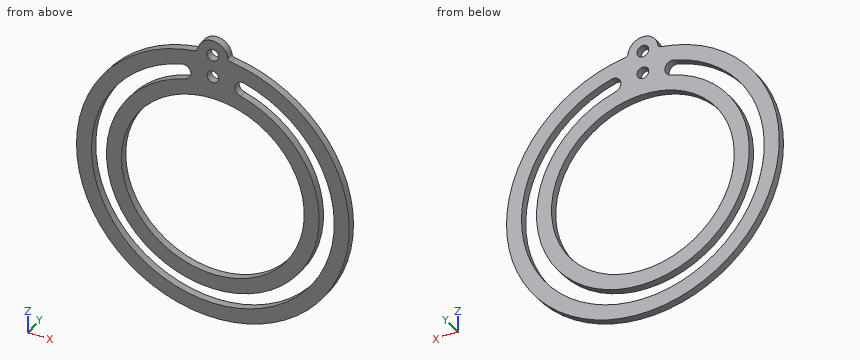
Autodesk Inventor part; units mm, degrees
ref_plane "YZ Plane" through (0, 0, 0) normal (1, 0, 0) x (0, 1, 0)
ref_plane "XZ Plane" through (0, 0, 0) normal (0, 1, 0) x (-1, 0, 0)
ref_plane "XY Plane" through (0, 0, 0) normal (0, 0, 1) x (1, 0, 0)
sketch "Sketch1" plane through (0, 0, 0) normal (0, 1, 0) x (-1, 0, 0)
  arc A0 (-9.3914, 47.3099) -> (9.3914, 47.3099) centre (0, 0) ccw
  arc A1 (-11.6619, 43.5227) -> (11.6619, 43.5227) centre (0, 0) ccw
  arc A2 (-13.3054, 49.6564) -> (13.3054, 49.6564) centre (0, 0) ccw
  circle A3 centre (0, 0) radius 38.708
  circle A4 centre (12.4836, 46.5895) radius 3.175
  circle A5 centre (-12.4836, 46.5895) radius 3.175
  line L0 (0, 0) -> (12.4836, 46.5895)
  line L1 (0, 0) -> (-12.4836, 46.5895)
  line L2 (0, 0) -> (0, 57.758)
  arc A6 (6.2927, 58.6092) -> (-6.2927, 58.6092) centre (0, 57.758) ccw
  arc A7 (6.2927, 58.6092) -> (7.6555, 57.2484) centre (7.8659, 58.8219) ccw
  arc A8 (-7.6555, 57.2484) -> (-6.2927, 58.6092) centre (-7.8659, 58.8219) ccw
  arc A9 (-7.6555, 57.2484) -> (7.6555, 57.2484) centre (0, 0) ccw
  point P0 (0, 48.233)
  point P1 (11.6619, 43.5227)
  point P2 (-11.6619, 43.5227)
  dimension "d0" = 96.4661
  dimension "d1" = 3.175
  dimension "d2" = 3.175
  dimension "d3" = 6.35
  dimension "d5" = 6.35
  dimension "d6" = 6.35
  dimension "d9" = 15
  dimension "d10" = 15
  dimension "d11" = 12.7
  dimension "d12" = 3.175
  dimension "d13" = 3.175
  dimension "d14" = 6.35
  dimension "d15" = 57.758
  dimension "d16" = 9.525
extrude "Extrusion1" add sketch "Sketch1" along normal blind 3.175 contours L1 A3 L0 A1 | A7 A9 A8 A6
hole "Hole1" at (0, 0, 48.233) at (0, 0, 57.758) direction (0, 1, 0) diameter 4.9784 end through all
equation "\"d0\" = ringDiam"
equation "\"d9\" = stageAngle"
equation "\"d10\" = stageAngle"
equation "\"d11\" = thickness"
equation "\"height\" = 203.2"
equation "\"thickness\" = 12.7"
equation "\"shaftDiam\" = 6.35"
equation "\"shaftSpace\" = 1.5875"
equation "\"stageSpace\" = 2.54"
equation "\"stageAngle\" = 15deg"
equation "\"bearingDiam\" = 9.5504"
equation "\"FlangeDiam\" = 12.7"
equation "\"FlangeDepth\" = 1.5875"
equation "\"smallFilet\" = 0.39687"
equation "\"ringDiam\" = 96.46608"
equation "\"stockHeight\" = 50.8"
equation "\"stockWidth\" = 76.2"
equation "\"stockRad\" = 9.525"
equation "\"stockGuage\" = 3.175"
equation "\"groundActu\" = 304.8"
equation "\"baseWidth\" = 1066.8"
equation "\"baseDepth\" = 254"
equation "\"capThickness\" = 3.175"
equation "\"sup1Len\" = 660.4"
equation "\"sup1Ang\" = 22.619865deg"
equation "\"sup2Len\" = 2079.37366"
equation "\"sup2Ang\" = 8.959949deg"
equation "\"supVertLen\" = 955.13561"
equation "\"supSideLen\" = 1531.12879"
equation "\"supSideAng\" = 19.376933deg"
properties part number "lock ring 2" material "Aluminum 6061"
Geometry: final body of the model. Coordinates: model frame, mm. Round coordinates to 2 decimals unless told otherwise and drop trailing zeros. Write each loop counter-clockwise with the first axis right and the second up, starting at its lowest first coordinate (ties: lowest second). Pieces come first, ordered by that corner, then holes.
Item 1: Pin query (flat end, axial travel): P1, Ø2, axis at x = -23, z = -28, coming from the +Y side; P2, Ø1.5, axis at x = 39, y = 1, coming from the +Z side. Return the tip coordinate at first contact, or that it passes through.
Item 2: Section query C-C (x = -15). Return loops of the section in (y, z) (3 decimals), plus the area to 3 significant figures.
Item 3: Section query B-B (x = 0). Return loops of the section in (y, z) (3 decimals), plus the area to 3 significant figures.
Item 4: Section query A-A (z = 0). Return loops of the section in (x, y) (3 decimals), plus the area to 3 significant figures.
Item 5: Section query D-D (y = 2.3). Give the number of separate pieces and of enclosed holes in the cut face, plus the area to 3 significant figures.
Item 6: Material intervals for L1, parallel to X at y = 1.55, z = 0; L2, parallel to Z at x = 1.5, y = 0.5; L3, parallel to X at y = 2.9, z = -21.5, sorted ascending.
Completed:
1. P1: passes through
1. P2: stops at z = 43.28
2. outline: (0, -55.776) - (3.175, -55.776) - (3.175, -49.171) - (0, -49.171) - close; (0, -42.488) - (3.175, -42.488) - (3.175, -35.683) - (0, -35.683) - close; (0, 35.683) - (3.175, 35.683) - (3.175, 42.488) - (0, 42.488) - close; (0, 49.171) - (3.175, 49.171) - (3.175, 55.776) - (0, 55.776) - close
2. area: 85.2 mm2
3. outline: (0, -57.758) - (3.175, -57.758) - (3.175, -51.408) - (0, -51.408) - close; (0, -45.058) - (3.175, -45.058) - (3.175, -38.708) - (0, -38.708) - close; (0, 38.708) - (3.175, 38.708) - (3.175, 45.744) - (0, 45.744) - close; (0, 50.722) - (3.175, 50.722) - (3.175, 55.269) - (0, 55.269) - close; (0, 60.247) - (3.175, 60.247) - (3.175, 64.108) - (0, 64.108) - close
3. area: 89.4 mm2
4. outline: (-57.758, 0) - (-51.408, 0) - (-51.408, 3.175) - (-57.758, 3.175) - close; (-45.058, 0) - (-38.708, 0) - (-38.708, 3.175) - (-45.058, 3.175) - close; (38.708, 0) - (45.058, 0) - (45.058, 3.175) - (38.708, 3.175) - close; (51.408, 0) - (57.758, 0) - (57.758, 3.175) - (51.408, 3.175) - close
4. area: 80.6 mm2
5. separate pieces: 1
5. enclosed holes: 4
5. area: 4,000 mm2
6. L1: x = -57.76 to -51.41, -45.06 to -38.71, 38.71 to 45.06, 51.41 to 57.76
6. L2: z = -57.74 to -51.39, -45.03 to -38.68, 38.68 to 46.25, 50.22 to 55.77, 59.74 to 63.93
6. L3: x = -53.61 to -46.7, -39.6 to -32.19, 32.19 to 39.6, 46.7 to 53.61
